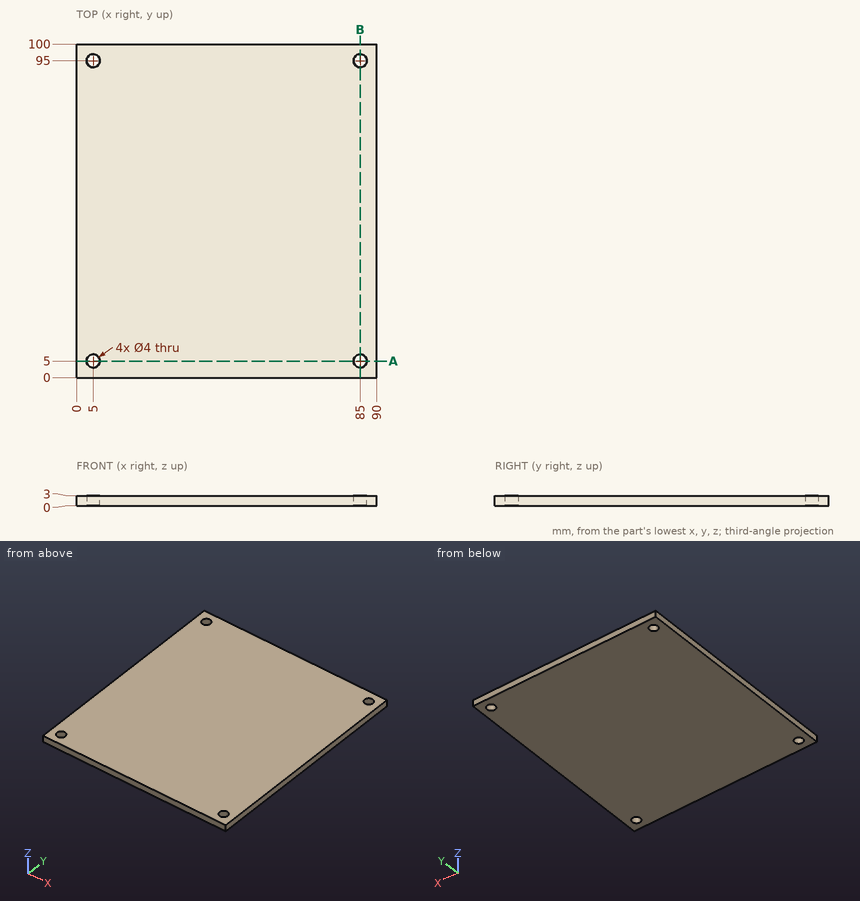
Input: dimensioned drawing with shaded views. Units: mm. Origin: part minimum x, y, z. Coordinates: 2 decimals unless noted, no trailing zeros. Loops run counter-clockwise (first coordinate to the right, second up) from the corner with the lowest first, then second, coordinate; pieces in that order, holes last. Notation, with made-up numbers: M 28.5,57 L 73.5,57 A18 ccw 73.5,78 Z; hole C 57.5,40.5 d7. An arc over 180 degrees is marked long. One line per item, written item: value.
(1) Line query: line 1 along Y through (x, z) = (5, 1.2); line 2 along X through (y, z) = (95, 0.7); line 3 along Y through (x, z) = (6.5, 1.75). Output: solid intervals per line, ascending. Write a range as from..to.
Filled in:
line 1: 0..3, 7..93, 97..100
line 2: 0..3, 7..83, 87..90
line 3: 0..3.68, 6.32..93.68, 96.32..100
(2) Section B-B (x = 85). Output: boundary loops of the cut face in (y, z), and give its area (3 significant figures).
Filled in:
outline: M 0,0 L 3,0 L 3,3 L 0,3 Z; M 7,0 L 93,0 L 93,3 L 7,3 Z; M 97,0 L 100,0 L 100,3 L 97,3 Z
area: 276 mm^2
(3) Section A-A (y = 5). Output: boundary loops of the cut face in (x, z).
Filled in:
outline: M 0,0 L 3,0 L 3,3 L 0,3 Z; M 7,0 L 83,0 L 83,3 L 7,3 Z; M 87,0 L 90,0 L 90,3 L 87,3 Z
